```python
from build123d import *

# Parameters (mm, degrees)
SKETCH1_R           = 3
BOSS_EXTRUDE1_DEPTH = 1.59


with BuildPart() as part:
    # Sketch1 → Boss-Extrude1 (new body)
    with BuildSketch(Plane.XY):
        with BuildLine():
            Line((5.147045903, 25.318285926), (6.030288505, 26.155519293))
            ThreePointArc((6.030288505, 26.155519293), (6.485334938, 26.402261945), (7.002788035, 26.388424134))
            ThreePointArc((7.002788035, 26.388424134), (12.054313697, 34.621489097), (3.563031664, 30.017208519))
            ThreePointArc((3.563031664, 30.017208519), (3.549193853, 29.499755422), (3.278483409, 29.058546801))
            Line((3.278483409, 29.058546801), (2.395240806, 28.221313434))
            ThreePointArc((2.395240806, 28.221313434), (1.940194374, 27.974570781), (1.422741277, 27.988408592))
            ThreePointArc((1.422741277, 27.988408592), (-4.593407333, 25.170095968), (-2.5, 18.864972981))
            ThreePointArc((-2.5, 18.864972981), (-2.133974596, 18.498947577), (-2, 17.998947577))
            Line((-2, 17.998947577), (-2, 5.766281297))
            ThreePointArc((-2, 5.766281297), (-2.145149586, 5.247406776), (-2.538461538, 4.879161098))
            ThreePointArc((-2.538461538, 4.879161098), (0, -5.5), (2.538461538, 4.879161098))
            ThreePointArc((2.538461538, 4.879161098), (2.145149586, 5.247406776), (2, 5.766281297))
            Line((2, 5.766281297), (2, 17.998947577))
            ThreePointArc((2, 17.998947577), (2.133974596, 18.498947577), (2.5, 18.864972981))
            ThreePointArc((2.5, 18.864972981), (4.593407333, 21.220104032), (4.862497647, 24.359624207))
            ThreePointArc((4.862497647, 24.359624207), (4.876335458, 24.877077304), (5.147045903, 25.318285926))
        make_face()
        Circle(SKETCH1_R, mode=Mode.SUBTRACT)
        with Locations((0, 23.1951)):
            Circle(SKETCH1_R, mode=Mode.SUBTRACT)
        with Locations((8.425529312, 31.181732726)):
            Circle(SKETCH1_R, mode=Mode.SUBTRACT)
    extrude(amount=BOSS_EXTRUDE1_DEPTH)


solid = part.part
```
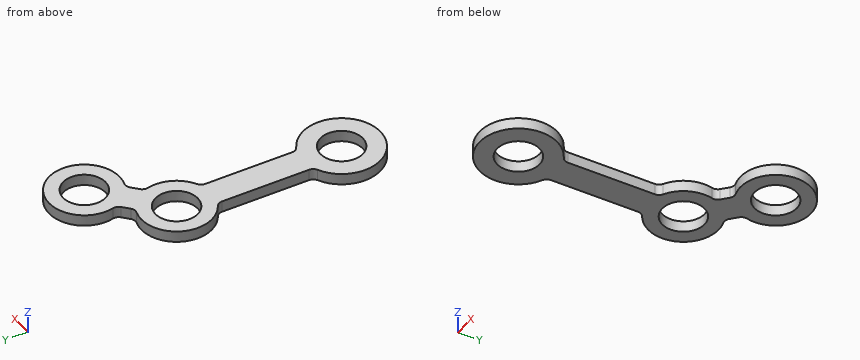
Geometry check sheet. Reference: the model listing, model coordinates, mm. Coordinates: 2 decimals unless noted, no trailing zeros. Order: outer loops, then holes, each group sorted by start corner. A loop starts at its lowest first (then second) coordinate and runs counter-clockwise, first axis right, second up. Notation, with made-up numbers: (84, 53) - (113, 53) arc R11 cw to (113, 70) - close; hole circle Ø10 at (45.5, 86). An arc over 180 degrees is marked (long way). Answer as a JSON object with one key per item and string values. Group by question number.
Item 1: Scan lines: probe 1 along Y at (x, z) = (-2.25, 1.15); probe 2 along X at (y, z) = (15, 0.55); probe 3 along Y at (x, z) = (8.5, 1.25). Record each from-to range of solid material in increasing order.
Item 2: Sectioned sample at D-D, the plane x = -4. Record the cut outline in (y, z), and give its area (3 significant figures).
Item 3: Sectioned sample at C-C, the plane z = 1.35. Record the cut outline in (x, y) (1 decimal).
Item 4: Sectioned sample at B-B, the plane y = 29.5. Record the cut outline in (x, z).
Item 5: Sectioned sample at A-A, the plane x = 0. Record the cut outline in (y, z).
Item 6: Depth check by flat-ended pin: pin 1 Ø5.5 at (x, y) = (0, 0) entering from -Z. Enter the tip coordinate at first touch or a pass-through.
Resolved:
{
 "1": {"probe 1": "-5.02 to -1.98, 1.98 to 5.1, 18.66 to 21.21, 25.18 to 27.66", "probe 2": "-2 to 2", "probe 3": "26.18 to 28.18, 34.18 to 36.18"},
 "2": {"outline": "(-3.77, 0) - (3.77, 0) - (3.77, 1.59) - (-3.77, 1.59) - close; (20.2, 0) - (26.2, 0) - (26.2, 1.59) - (20.2, 1.59) - close", "area": "21.5 mm^2"},
 "3": {"outline": "(-2.5, 4.9) arc R5.5 ccw (long way) to (2.5, 4.9) arc R1 cw to (2, 5.8) - (2, 18) arc R1 cw to (2.5, 18.9) arc R5 ccw to (4.9, 24.4) arc R1 cw to (5.1, 25.3) - (6, 26.2) arc R1 cw to (7, 26.4) arc R5 ccw (long way) to (3.6, 30) arc R1 cw to (3.3, 29.1) - (2.4, 28.2) arc R1 cw to (1.4, 28) arc R5 ccw to (-2.5, 18.9) arc R1 cw to (-2, 18) - (-2, 5.8) arc R1 cw to start; hole circle Ø6 at (0, 0); hole circle Ø6 at (0, 23.2); hole circle Ø6 at (8.4, 31.2)"},
 "4": {"outline": "(3.55, 0) - (5.94, 0) - (5.94, 1.59) - (3.55, 1.59) - close; (10.91, 0) - (13.13, 0) - (13.13, 1.59) - (10.91, 1.59) - close"},
 "5": {"outline": "(-5.5, 0) - (-3, 0) - (-3, 1.59) - (-5.5, 1.59) - close; (3, 0) - (20.2, 0) - (20.2, 1.59) - (3, 1.59) - close; (26.2, 0) - (28.2, 0) - (28.2, 1.59) - (26.2, 1.59) - close"},
 "6": {"pin 1": "through"}
}
